```python
from build123d import *

# Parameters (mm, degrees)
PAD_DEPTH       = 11
FILLET_R        = 1
FILLET001_R     = 1
SKETCH001_W     = 5
SKETCH001_H     = 11
PAD001_DEPTH    = 20
SKETCH002_W     = 20
SKETCH002_H     = 5
PAD002_DEPTH    = 20
SKETCH003_R     = 5
POCKET_DEPTH    = 3.3
PAD003_DEPTH    = 5
SKETCH005_R     = 2.5
POCKET001_DEPTH = 5
FILLET002_R     = 2


with BuildPart() as part:
    # Sketch → Pad (new body)
    with BuildSketch(Plane.XZ):
        with BuildLine():
            Line((0, 0), (0, 20))
            Line((0, 20), (-3, 20))
            Line((-3, 20), (-3, 15))
            ThreePointArc((-3, 15), (-11.080706, 18.723006), (-19.399163, 15.566764))
            Line((-17.330276, 13.868571), (-19.399163, 15.566764))
            ThreePointArc((-18.108729, 1.368571), (-2.645027, 6.679789), (-17.330276, 13.868571))
            Line((-18.108729, 1.368571), (-20.421014, 0))
            ThreePointArc((-20.421014, 0), (-15.279185, -3.623719), (-9, -4))
            Line((-9, -4), (0, -4))
            Line((0, 0), (0, -4))
        make_face()
    extrude(amount=PAD_DEPTH)

    # Fillet
    fillet_edges = [part.edges().sort_by_distance(p)[0] for p in [
        (-18.108729, -5.5, 1.368571),
        (-20.421014, -5.5, 0),
        (-19.264872, 0, 0.684285),
        (-19.264872, -11, 0.684285),
    ]]
    fillet(fillet_edges, radius=FILLET_R)

    # Fillet001
    fillet001_edges = [part.edges().sort_by_distance(p)[0] for p in [
        (-17.330276, -5.5, 13.868571),
        (-19.399163, -5.5, 15.566764),
        (-18.364719, 0, 14.717668),
        (-18.364719, -11, 14.717668),
    ]]
    fillet(fillet001_edges, radius=FILLET001_R)

    # Sketch001 (on Face17 of Fillet001) → Pad001 (join)
    with BuildSketch(Plane(origin=(0, 0, 0), x_dir=(0, 0, 1), z_dir=(1, 0, 0))):
        with Locations((-1.5, 5.5)):
            Rectangle(SKETCH001_W, SKETCH001_H)
    extrude(amount=PAD001_DEPTH)

    # Sketch002 (on Face21 of Pad001) → Pad002 (join)
    with BuildSketch(Plane.XZ.offset(11)):
        with Locations((10, -1.5)):
            Rectangle(SKETCH002_W, SKETCH002_H)
    extrude(amount=PAD002_DEPTH)

    # Sketch003 (on Face26 of Pad002) → Pocket (cut)
    with BuildSketch(Plane(origin=(0, 0, -4), x_dir=(1, 0, 0), z_dir=(0, 0, -1))):
        with Locations((10, 23)):
            Circle(SKETCH003_R)
        with Locations((10, 8)):
            Circle(SKETCH003_R)
    extrude(amount=-POCKET_DEPTH, mode=Mode.SUBTRACT)

    # Sketch004 (on Face15 of Pocket) → Pad003 (join)
    with BuildSketch(Plane(origin=(0, 0, -4), x_dir=(1, 0, 0), z_dir=(0, 0, -1))):
        with BuildLine():
            ThreePointArc((-5, 11), (-1.464466, 12.464466), (0, 16))
            Line((0, 16), (0, 11))
            Line((0, 11), (-5, 11))
        make_face()
    extrude(amount=-PAD003_DEPTH)

    # Sketch005 (on Face35 of Pad003) → Pocket001 (cut)
    with BuildSketch(Plane(origin=(0, 0, -0.7), x_dir=(1, 0, 0), z_dir=(0, 0, -1))):
        with Locations((10, 23)):
            Circle(SKETCH005_R)
        with Locations((10, 8)):
            Circle(SKETCH005_R)
    extrude(amount=-POCKET001_DEPTH, mode=Mode.SUBTRACT)

    # Fillet002
    fillet002_edges = [part.edges().sort_by_distance(p)[0] for p in [
        (10, -31, -4),
        (20, -21, -4),
        (10, 0, -4),
        (20, -5.5, -4),
    ]]
    fillet(fillet002_edges, radius=FILLET002_R)


solid = part.part
```
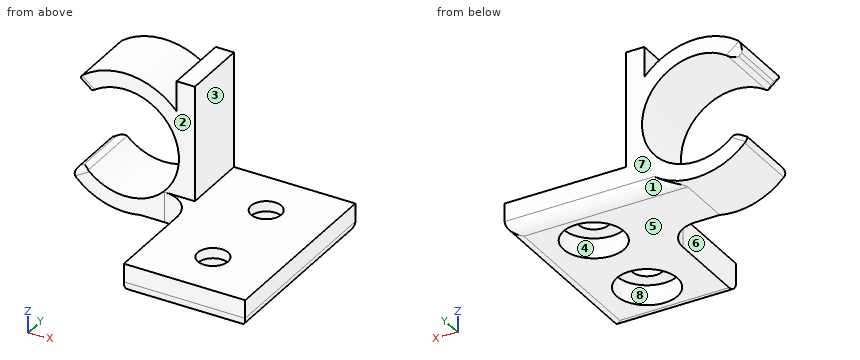
Geometry: final body of the model. Coordinates: model frame, mm. Face numbers are marked on the shaded views. A direction names the side the tool comes from. Give positions to 0.01 mm unless a question says otherwise; leave off trailing zeros. Write each loop counter-clockwise with the first axis right and the second up, starting at its lowest first coordinate (ties: lowest second). Pieces come first, ordered by that corner, then holes.
1. Draft query along X for the marked faces 6, 7 and 8. Return one class per face: released by +X, released by -X, zero draft, split by the parting line, or undercut.
2. Section query C-C, the plane y = -19. Return loops of the section in (x, z).
3. Section query B-B, the plane x = 10. Return loops of the section in (y, z), then the cut area to 3 significant figures.
4. Pin query (flat end, axial travel): P1, Ø11, axis at x = 8.5, y = -24.5, coming from the -Z side; P2, Ø1, axis at x = 6.5, y = -16, coming from the +Z side; P3, Ø2.5, axis at y = -20, z = -2.5, coming from the -X side. Return the tip coordinate at first contact, or that it passes through.
5. Reachability of the marked faces 1, 2, 3, 4 and 5 from +Z, -Z, +X, -X, +Y, -Y: full face, straight path, thin tool, end or side. Return the list, or none.
6. Section query D-D, the plane x = 2. Return loops of the section in (y, z).
7. Line query: probe 1 along Y at (x, z) = (10, -1.8); probe 2 along Y at (x, z) = (10, -0.2); probe 3 along X at (y, z) = (-8, 0.1). Output: solid intervals per line, ascending.
8. Section query A-A, the plane y = -23. Return loops of the section in (x, z).
Computed:
1. face 6: released by -X
1. face 7: zero draft
1. face 8: undercut
2. outline: (0, -4) - (7, -4) - (7, -0.7) - (13, -0.7) - (13, -4) - (18, -4) arc R2 ccw to (20, -2) - (20, 1) - (0, 1) - close
3. outline: (-31, -2) arc R2 ccw to (-29, -4) - (-28, -4) - (-28, -0.7) - (-25.5, -0.7) - (-25.5, 1) - (-31, 1) - close; (-20.5, -0.7) - (-18, -0.7) - (-18, -4) - (-13, -4) - (-13, -0.7) - (-10.5, -0.7) - (-10.5, 1) - (-20.5, 1) - close; (-5.5, -0.7) - (-3, -0.7) - (-3, -4) - (-2, -4) arc R2 ccw to (0, -2) - (0, 1) - (-5.5, 1) - close
3. area: 70.3 mm2
4. P1: stops at z = -4
4. P2: stops at z = 1
4. P3: stops at x = 0
5. face 1: -Z, +X, +Y
5. face 2: +Z, -X, -Y
5. face 3: +Z, +X, +Y, -Y
5. face 4: -Z
5. face 5: -Z, +X, +Y, -Y
6. outline: (-31, -2) arc R2 ccw to (-29, -4) - (-2, -4) arc R2 ccw to (0, -2) - (0, 1) - (-31, 1) - close
7. probe 1: y = -31 to -28, -18 to -13, -3 to 0
7. probe 2: y = -31 to -25.5, -20.5 to -10.5, -5.5 to 0
7. probe 3: x = -19.8 to -16.72, -6.24 to 7.5, 12.5 to 20
8. outline: (0, -4) - (5, -4) - (5, -0.7) - (7.5, -0.7) - (7.5, 1) - (0, 1) - close; (12.5, -0.7) - (15, -0.7) - (15, -4) - (18, -4) arc R2 ccw to (20, -2) - (20, 1) - (12.5, 1) - close
